The model under review builds one solid part; all positions refer to its coordinate system, in mm. A direction names the side the tool comes from. Round coordinates to 2 decimals unless told otherwise and drop trailing zeros. Order: outer loops, then holes, each group sorted by start corner. A loop starts at its lowest first (then second) coordinate and runs counter-clockwise, first axis right, second up. Notation, with made-up numbers: M 65.25,21 L 81.25,21 A32 ccw 81.25,59 Z; hole C 6.25,86 d2. An arc over 180 degrees is marked long. Answer as a JSON object with one key per item and string values. Group by question number.
1) Consider section A-A, the plane y = 1.05. Write out the cut boundary in (x, z), then the cut area to 3 significant figures.
2) For faces 4 (the flat face through (0.3, 1.5, 0.5)), 5 (the flat face through (-0.3, -1.5, 0.5)), 6 (the cylindrical face through (23.477, 0.15, 0.493)), 7 (the flat face through (24, 0, 1)), list the 3-axis set-ups (+Z, -Z, +X, -X, +Y, -Y) from which the entire face can be reached by the end or side of a thin tool; tool diameter is ignored.
3) The part is to be moulded in two halves that separate along X. For faces 1 (the cylindrical face through (-25, 0, 1)), 2 (the cylindrical face through (25, 0, 1)), 3 (the flat face through (0, 0, 0)), say which applies: +X half, -X half, draft (parallel to the pull), parting line (faces both ways), or undercut.
4) Consider section B-B, the plane x = 19. Write out the cut boundary in (y, z), then the cut area to 3 significant figures.
5) Insertion check: pin 1 Ø0.9 at (x, y) = (10.5, -0.5) entering from +Z. The pin has a flat end and moves straight along its axis. Give the tip position at first contact, or say it passes through.
6) To check wall thickness, follow line 1 (Y direction, x = -23, z = 0.85); line 2 (Z direction, x = -19.5, y = 0.25); line 3 (Y direction, x = -16, z = 0.9). State the ranges of each line that lie inside material, in increasing order.
```python
from build123d import *

# Parameters (mm, degrees)
F0_R     = 0.5
F1_DEPTH = 1
F2_DEPTH = 1.4


with BuildPart() as f1:
    # F0 (on Top) → F1 (new body)
    with BuildSketch(Plane.XY):
        with BuildLine():
            ThreePointArc((-23, 1.5), (-24.5, 0), (-23, -1.5))
            ThreePointArc((-23, -1.5), (-21.9393398282, -1.0606601718), (-21.5, 0))
            ThreePointArc((-21.5, 0), (-21.9393398282, 1.0606601718), (-23, 1.5))
        make_face()
        with Locations((-23, 0)):
            Circle(F0_R, mode=Mode.SUBTRACT)
        with BuildLine():
            Line((-23, -1.5), (-24.3228756555, -1.5))
            ThreePointArc((-24.3228756555, -1.5), (-23, -2), (-21.6771243445, -1.5))
            Line((-21.6771243445, -1.5), (-23, -1.5))
        make_face()
        with BuildLine():
            ThreePointArc((-21.6771243445, 1.5), (-23, 2), (-24.3228756555, 1.5))
            Line((-24.3228756555, 1.5), (-23, 1.5))
            Line((-23, 1.5), (-21.6771243445, 1.5))
        make_face()
        with BuildLine():
            ThreePointArc((-21, 0), (-21.1771243445, -0.8228756555), (-21.6771243445, -1.5))
            Line((-21.6771243445, -1.5), (21.6771243445, -1.5))
            ThreePointArc((21.6771243445, -1.5), (21, 0), (21.6771243445, 1.5))
            Line((21.6771243445, 1.5), (-21.6771243445, 1.5))
            ThreePointArc((-21.6771243445, 1.5), (-21.1771243445, 0.8228756555), (-21, 0))
        make_face()
        with BuildLine():
            ThreePointArc((23, 1.5), (21.5, 0), (23, -1.5))
            ThreePointArc((23, -1.5), (24.0606601718, -1.0606601718), (24.5, 0))
            ThreePointArc((24.5, 0), (24.0606601718, 1.0606601718), (23, 1.5))
        make_face()
        with Locations((23, 0)):
            Circle(F0_R, mode=Mode.SUBTRACT)
        with BuildLine():
            Line((23, -1.5), (21.6771243445, -1.5))
            ThreePointArc((21.6771243445, -1.5), (23, -2), (24.3228756555, -1.5))
            Line((24.3228756555, -1.5), (23, -1.5))
        make_face()
        with BuildLine():
            ThreePointArc((24.3228756555, 1.5), (23, 2), (21.6771243445, 1.5))
            Line((21.6771243445, 1.5), (23, 1.5))
            Line((23, 1.5), (24.3228756555, 1.5))
        make_face()
        with BuildLine():
            ThreePointArc((21.6771243445, 1.5), (21, 0), (21.6771243445, -1.5))
            Line((21.6771243445, -1.5), (23, -1.5))
            ThreePointArc((23, -1.5), (21.5, 0), (23, 1.5))
            Line((23, 1.5), (21.6771243445, 1.5))
        make_face()
        with BuildLine():
            ThreePointArc((24.5, 0), (24.0606601718, -1.0606601718), (23, -1.5))
            Line((23, -1.5), (24.3228756555, -1.5))
            ThreePointArc((24.3228756555, -1.5), (24.8228756555, -0.8228756555), (25, 0))
            ThreePointArc((25, 0), (24.8228756555, 0.8228756555), (24.3228756555, 1.5))
            Line((24.3228756555, 1.5), (23, 1.5))
            ThreePointArc((23, 1.5), (24.0606601718, 1.0606601718), (24.5, 0))
        make_face()
        with BuildLine():
            ThreePointArc((-25, 0), (-24.8228756555, -0.8228756555), (-24.3228756555, -1.5))
            Line((-24.3228756555, -1.5), (-23, -1.5))
            ThreePointArc((-23, -1.5), (-24.5, 0), (-23, 1.5))
            Line((-23, 1.5), (-24.3228756555, 1.5))
            ThreePointArc((-24.3228756555, 1.5), (-24.8228756555, 0.8228756555), (-25, 0))
        make_face()
        with BuildLine():
            ThreePointArc((-21.5, 0), (-21.9393398282, -1.0606601718), (-23, -1.5))
            Line((-23, -1.5), (-21.6771243445, -1.5))
            ThreePointArc((-21.6771243445, -1.5), (-21.1771243445, -0.8228756555), (-21, 0))
            ThreePointArc((-21, 0), (-21.1771243445, 0.8228756555), (-21.6771243445, 1.5))
            Line((-21.6771243445, 1.5), (-23, 1.5))
            ThreePointArc((-23, 1.5), (-21.9393398282, 1.0606601718), (-21.5, 0))
        make_face()
    extrude(amount=F1_DEPTH)

    # F0 (on Top) → F2 (join)
    with BuildSketch(Plane.XY):
        with BuildLine():
            Line((-23, -1.5), (-24.3228756555, -1.5))
            ThreePointArc((-24.3228756555, -1.5), (-23, -2), (-21.6771243445, -1.5))
            Line((-21.6771243445, -1.5), (-23, -1.5))
        make_face()
        with BuildLine():
            ThreePointArc((-25, 0), (-24.8228756555, -0.8228756555), (-24.3228756555, -1.5))
            Line((-24.3228756555, -1.5), (-23, -1.5))
            ThreePointArc((-23, -1.5), (-24.5, 0), (-23, 1.5))
            Line((-23, 1.5), (-24.3228756555, 1.5))
            ThreePointArc((-24.3228756555, 1.5), (-24.8228756555, 0.8228756555), (-25, 0))
        make_face()
        with BuildLine():
            ThreePointArc((-21.5, 0), (-21.9393398282, -1.0606601718), (-23, -1.5))
            Line((-23, -1.5), (-21.6771243445, -1.5))
            ThreePointArc((-21.6771243445, -1.5), (-21.1771243445, -0.8228756555), (-21, 0))
            ThreePointArc((-21, 0), (-21.1771243445, 0.8228756555), (-21.6771243445, 1.5))
            Line((-21.6771243445, 1.5), (-23, 1.5))
            ThreePointArc((-23, 1.5), (-21.9393398282, 1.0606601718), (-21.5, 0))
        make_face()
        with BuildLine():
            ThreePointArc((-21.6771243445, 1.5), (-23, 2), (-24.3228756555, 1.5))
            Line((-24.3228756555, 1.5), (-23, 1.5))
            Line((-23, 1.5), (-21.6771243445, 1.5))
        make_face()
        with BuildLine():
            Line((23, -1.5), (21.6771243445, -1.5))
            ThreePointArc((21.6771243445, -1.5), (23, -2), (24.3228756555, -1.5))
            Line((24.3228756555, -1.5), (23, -1.5))
        make_face()
        with BuildLine():
            ThreePointArc((24.5, 0), (24.0606601718, -1.0606601718), (23, -1.5))
            Line((23, -1.5), (24.3228756555, -1.5))
            ThreePointArc((24.3228756555, -1.5), (24.8228756555, -0.8228756555), (25, 0))
            ThreePointArc((25, 0), (24.8228756555, 0.8228756555), (24.3228756555, 1.5))
            Line((24.3228756555, 1.5), (23, 1.5))
            ThreePointArc((23, 1.5), (24.0606601718, 1.0606601718), (24.5, 0))
        make_face()
        with BuildLine():
            ThreePointArc((24.3228756555, 1.5), (23, 2), (21.6771243445, 1.5))
            Line((21.6771243445, 1.5), (23, 1.5))
            Line((23, 1.5), (24.3228756555, 1.5))
        make_face()
        with BuildLine():
            ThreePointArc((21.6771243445, 1.5), (21, 0), (21.6771243445, -1.5))
            Line((21.6771243445, -1.5), (23, -1.5))
            ThreePointArc((23, -1.5), (21.5, 0), (23, 1.5))
            Line((23, 1.5), (21.6771243445, 1.5))
        make_face()
    extrude(amount=F2_DEPTH)


solid = f1.part
```
Results list:
{
 "1": {"outline": "M -24.7,0 L 24.7,0 L 24.7,1.4 L 24.07,1.4 L 24.07,1 L 21.93,1 L 21.93,1.4 L 21.3,1.4 L 21.3,1 L -21.3,1 L -21.3,1.4 L -21.93,1.4 L -21.93,1 L -24.07,1 L -24.07,1.4 L -24.7,1.4 Z", "area": "50.4 mm^2"},
 "2": {"face 4": "+Z, -Z, +Y", "face 5": "+Z, -Z, -Y", "face 6": "+Z, -Z", "face 7": "+Z"},
 "3": {"face 1": "undercut", "face 2": "undercut", "face 3": "draft"},
 "4": {"outline": "M -1.5,0 L 1.5,0 L 1.5,1 L -1.5,1 Z", "area": "3.00 mm^2"},
 "5": {"pin 1": "z = 1"},
 "6": {"line 1": "-2 to -0.5, 0.5 to 2", "line 2": "0 to 1", "line 3": "-1.5 to 1.5"}
}
